Verification items for this drawing (mm, ordinates from the low corner). A direction names the side the tool comes from. Round coordinates to 2 decimals unless told otherwise and drop trailing zeros. Order: outer loops, then holes, each group sorted by start corner. A loop starts at its lowest first (then second) coordinate and runs counter-clockwise, first axis right, second up.
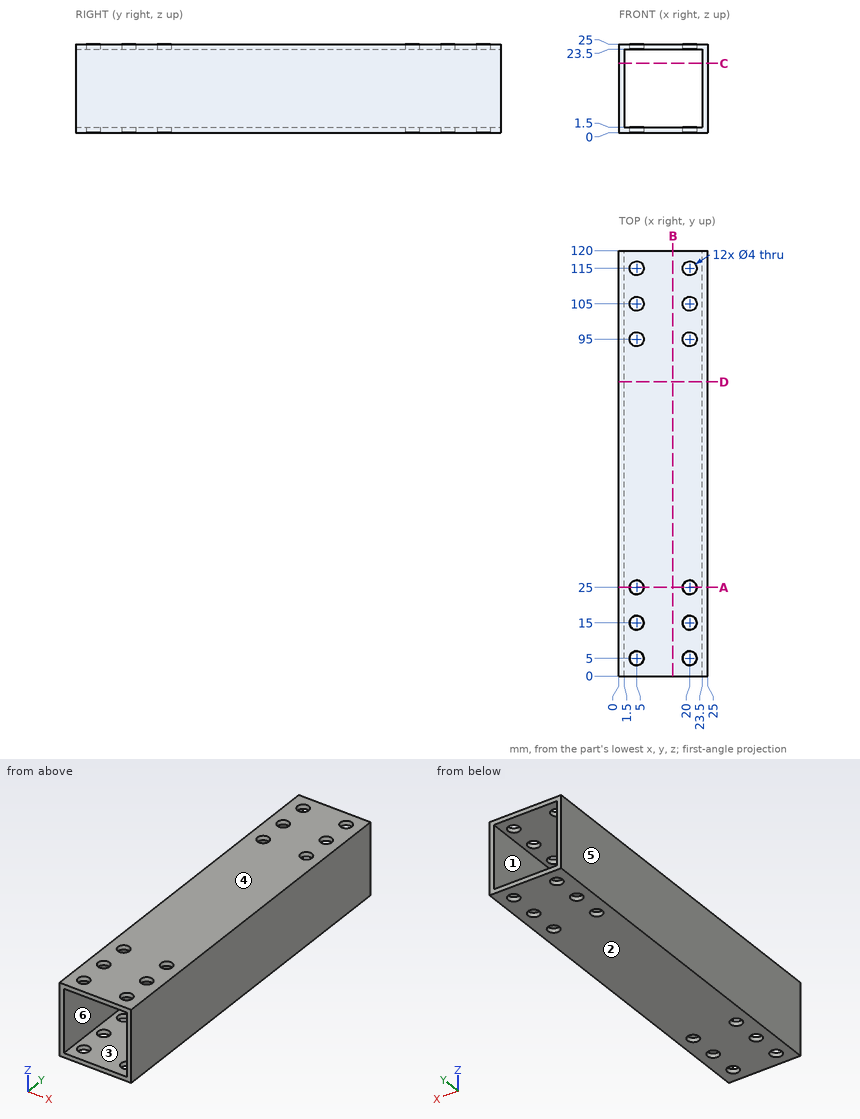
Item 1: Go/stop test with a flat-tipped pin: P1, Ø3.5, axis at x = 20, y = 25, coming from the -Z side. Record where the tip stops, or that it passes through.
Answer:
P1: passes through
Item 2: Sectioned sample at A-A (y = 25). Record the cut outline in (x, z).
Answer:
outline: (0, 0) - (3, 0) - (3, 1.5) - (1.5, 1.5) - (1.5, 23.5) - (3, 23.5) - (3, 25) - (0, 25) - close; (7, 0) - (18, 0) - (18, 1.5) - (7, 1.5) - close; (7, 23.5) - (18, 23.5) - (18, 25) - (7, 25) - close; (22, 0) - (25, 0) - (25, 25) - (22, 25) - (22, 23.5) - (23.5, 23.5) - (23.5, 1.5) - (22, 1.5) - close
Item 3: Sectioned sample at D-D (y = 83). Record the cut outline in (x, z).
Answer:
outline: (0, 0) - (25, 0) - (25, 25) - (0, 25) - close; hole (1.5, 1.5) - (23.5, 1.5) - (23.5, 23.5) - (1.5, 23.5) - close
Item 4: Sectioned sample at B-B (x = 15.25). Record the cut outline in (y, z).
Answer:
outline: (0, 0) - (120, 0) - (120, 1.5) - (0, 1.5) - close; (0, 23.5) - (120, 23.5) - (120, 25) - (0, 25) - close
Item 5: Access from +Z, -Z, +X, -X, +Y, -Y to the whole of each face (thin tool, end or side, straight path). Record for the marked faces 5 and 6.
Answer:
face 5: +Z, -Z, -X, +Y, -Y
face 6: +Y, -Y
Item 6: Sectioned sample at C-C (z = 19.5). Record the cut outline in (x, y).
Answer:
outline: (0, 0) - (1.5, 0) - (1.5, 120) - (0, 120) - close; (23.5, 0) - (25, 0) - (25, 120) - (23.5, 120) - close
Item 7: Scan lines: line 1 along X through (y, z) = (95, 24.6); line 2 along X through (y, z) = (15.5, 14). Record each from-to range of solid material in increasing order.
Answer:
line 1: x = 0 to 3, 7 to 18, 22 to 25
line 2: x = 0 to 1.5, 23.5 to 25
Item 8: Release check for a two-part mould opening along Z. For the marked faces 1, 2, 3 and 4 record: released by +Z, released by -Z, zero draft, split by the parting line, or undercut.
Answer:
face 1: undercut
face 2: released by -Z
face 3: undercut
face 4: released by +Z
